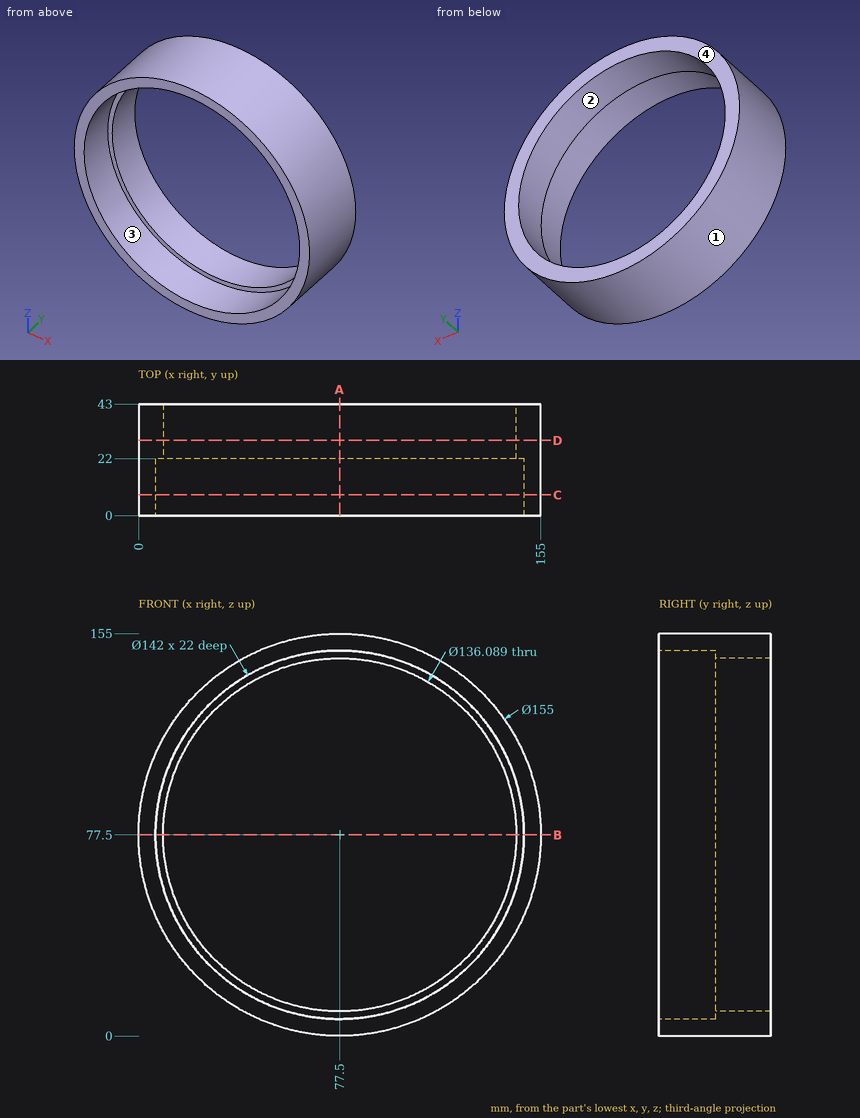
Source: three-view drawing plus pictorial views. Frame: mm from the lowest corner of the part. Round coordinates to 2 decimals unless told otherwise and drop trailing zeros. Loops run counter-clockwise (first coordinate to the right, second up) from the corner with the lowest first, then second, coordinate; pieces in that order, holes last. Notation, with made-up numbers: M 38.25,-34 L 75.25,-34 A30 cw 75.25,-10 Z; hole C 14.5,84.25 d1. An arc over 180 degrees is marked long. Answer as CSV lines item,"result".
Q1. Pull-direction query (X, two-part tool) for the marked faces 1, 2, 3 and 4; classes: +X half, -X half, draft (parallel to the pull), parting line (faces both ways), or undercut.
Verdict:
face 1,"parting line"
face 2,"undercut"
face 3,"undercut"
face 4,"draft"
Q2. Cut plane C-C (y = 8). Return the cut outline in (x, z).
Verdict:
outline,"C 77.5,77.5 d155; hole C 77.5,77.5 d142"
Q3. Line query: line 1 along Z through (x, y) = (77.5, 8.25); line 2 along X through (y, z) = (35, 77.5) (1 decimal). Output: solid intervals per line, ascending.
Verdict:
line 1,"z = 0 to 6.5, 148.5 to 155"
line 2,"x = 0 to 9.5, 145.5 to 155"
Q4. Cut plane A-A (x = 77.5). Return the cut outline in (y, z) (1 decimal), plus the area to 3 significant figures.
Verdict:
outline,"M 0,0 L 43,0 L 43,9.5 L 22,9.5 L 22,6.5 L 0,6.5 Z; M 0,148.5 L 22,148.5 L 22,145.5 L 43,145.5 L 43,155 L 0,155 Z"
area,"683 mm^2"
Q5. Contact query for flat-ended pins moving along their axis: pin 1 (8 mm diameter, centred on x = 30.5, z = 33, fed in from +Y); pin 2 (3 mm diameter, centred on x = 88, y = 32.5, fed in from -Z); pin 3 (2 mm diameter, centred on x = 39.5, y = 31, fed in from +Z); pin 4 (3 mm diameter, centred on x = 139, y = 23.5, fed in from -Z) (1 decimal). Output: stop coordinate, or through.
Verdict:
pin 1,"stops at y = 43"
pin 2,"stops at z = 0.52"
pin 3,"stops at z = 145.6"
pin 4,"stops at z = 28.4"
Q6. Cut plane D-D (y = 29). Return the cut outline in (x, z) (1 decimal), plus the area to 3 significant figures.
Verdict:
outline,"C 77.5,77.5 d155; hole C 77.5,77.5 d136.1"
area,"4,320 mm^2"
Q7. Cut plane B-B (z = 77.5). Return the cut outline in (x, y) (1 decimal).
Verdict:
outline,"M 0,0 L 6.5,0 L 6.5,22 L 9.5,22 L 9.5,43 L 0,43 Z; M 145.5,22 L 148.5,22 L 148.5,0 L 155,0 L 155,43 L 145.5,43 Z"
